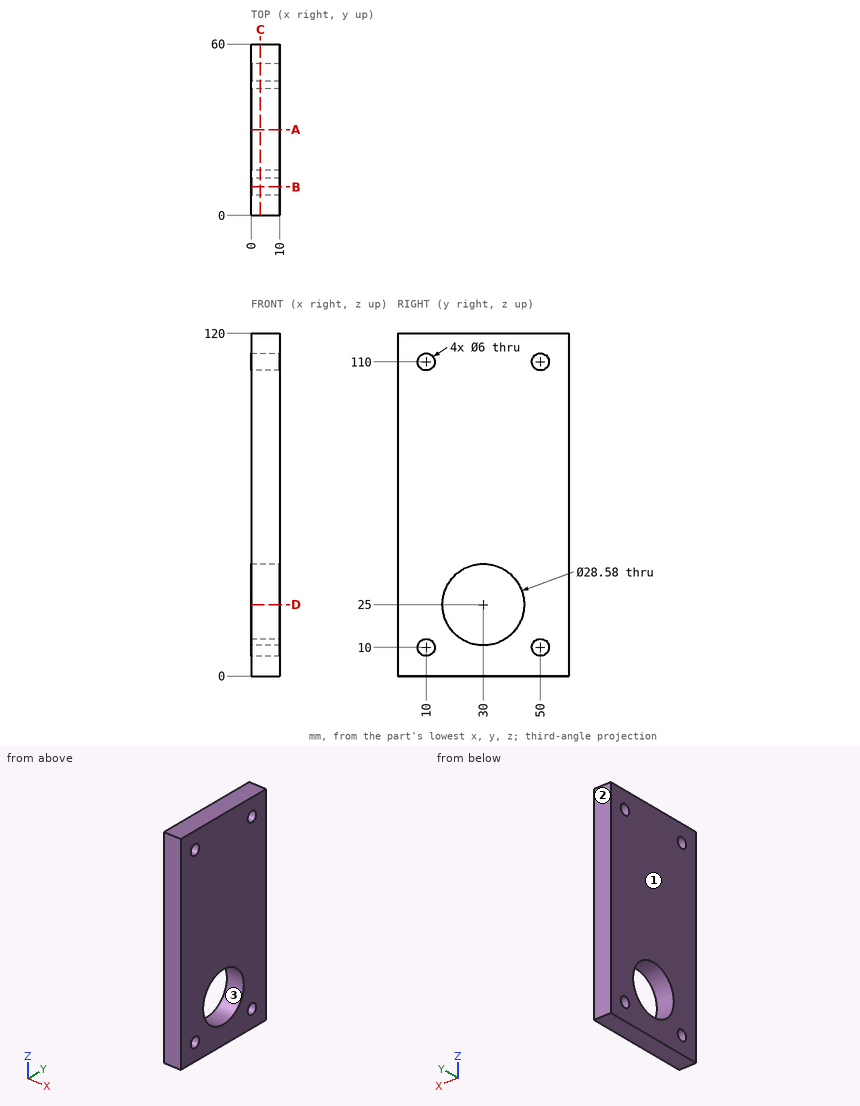
The figure shows three views and two pictorial views of one solid part (mm, origin at its lowest corner). Answer the questions. Round coordinates to 2 decimals unless told otherwise and drop trailing zeros. Order: outer loops, then holes, each group sorted by start corner. A loop starts at its lowest first (then second) coordinate and runs counter-clockwise, first axis right, second up. Notation, with made-up numbers: (-1.75, 66.25) -> (10.25, 66.25) arc R27 ccw to (10.25, 85.25) -> close; hole circle Ø8 at (-32, 77.5). An arc over 180 degrees is marked (long way). Put each result on its own line as item: value.
Q1. Section D-D, the plane z = 25 is taken. Write down the section's boundary in (x, y), and give its area (3 significant figures).
Results list:
outline: (0, 0) -> (10, 0) -> (10, 15.71) -> (0, 15.71) -> close; (0, 44.29) -> (10, 44.29) -> (10, 60) -> (0, 60) -> close
area: 314 mm^2
Q2. Section C-C, the plane x = 3.25 is taken. Write down the section's boundary in (y, z), and give its area (3 significant figures).
Results list:
outline: (0, 0) -> (60, 0) -> (60, 120) -> (0, 120) -> close; hole circle Ø6 at (10, 10); hole circle Ø6 at (10, 110); hole circle Ø28.58 at (30, 25); hole circle Ø6 at (50, 10); hole circle Ø6 at (50, 110)
area: 6,450 mm^2
Q3. Section B-B, the plane y = 10 is taken. Write down the section's boundary in (x, z).
Results list:
outline: (0, 0) -> (10, 0) -> (10, 7) -> (0, 7) -> close; (0, 13) -> (10, 13) -> (10, 107) -> (0, 107) -> close; (0, 113) -> (10, 113) -> (10, 120) -> (0, 120) -> close
Q4. Determine the mould class of the marked faces 1, 2 and 3 for opening direction Y: pulls with the +Y half, pulls with the -Y half, needs draft (parallel to the pull), parting line crosses it, or undercut.
Results list:
face 1: needs draft
face 2: pulls with the +Y half
face 3: undercut
Q5. Section A-A, the plane y = 30 is taken. Write down the section's boundary in (x, z).
Results list:
outline: (0, 0) -> (10, 0) -> (10, 10.71) -> (0, 10.71) -> close; (0, 39.29) -> (10, 39.29) -> (10, 120) -> (0, 120) -> close
Q6. Consider line 1 along Y through (x, z) = (5.75, 10); line 2 along Y through (x, z) = (5, 108.5); line 3 along Z through (x, y) = (5, 40). Determine where each line is inside the solid, lowest interval first.
Results list:
line 1: 0 to 7, 13 to 47, 53 to 60
line 2: 0 to 7.4, 12.6 to 47.4, 52.6 to 60
line 3: 0 to 14.79, 35.21 to 120
